```python
from build123d import *

# Parameters (mm, degrees)
F0_W     = 31.8
F0_H     = 15.8
F1_DEPTH = 9.6
F2_R     = 2.4
F3_DEPTH = 1.8
F4_W     = 29.4
F4_H     = 13.4
F5_DEPTH = 8.4
F5_TAPER = 1.5
F6_R     = 1.3
F7_DEPTH = 1.7
F8_R     = 3.25
F8_R_2   = 2.4
F9_DEPTH = 8.4


with BuildPart() as f1:
    # F0 (on Top) → F1 (new body)
    with BuildSketch(Plane.XY):
        Rectangle(F0_W, F0_H)
    extrude(amount=F1_DEPTH)

    # F2 (on face) → F3 (join)
    with BuildSketch(Plane.XY.offset(9.6)):
        with Locations((-12, 4)):
            Circle(F2_R)
        with Locations((-12, -4)):
            Circle(F2_R)
        with Locations((-4, 4)):
            Circle(F2_R)
        with Locations((-4, -4)):
            Circle(F2_R)
        with Locations((4, 4)):
            Circle(F2_R)
        with Locations((4, -4)):
            Circle(F2_R)
        with Locations((12, 4)):
            Circle(F2_R)
        with Locations((12, -4)):
            Circle(F2_R)
    extrude(amount=F3_DEPTH)

    # F4 (on face) → F5 (cut)
    with BuildSketch(Plane(origin=(0, 0, 0), x_dir=(1, 0, 0), z_dir=(0, 0, -1))):
        Rectangle(F4_W, F4_H)
    extrude(amount=-F5_DEPTH, taper=F5_TAPER, mode=Mode.SUBTRACT)

    # F6 (on face) → F7 (cut)
    with BuildSketch(Plane(origin=(0, 0, 8.4), x_dir=(1, 0, 0), z_dir=(0, 0, -1))):
        with Locations((-12, 4)):
            Circle(F6_R)
        with Locations((-4, 4)):
            Circle(F6_R)
        with Locations((4, 4)):
            Circle(F6_R)
        with Locations((12, 4)):
            Circle(F6_R)
        with Locations((12, -4)):
            Circle(F6_R)
        with Locations((4, -4)):
            Circle(F6_R)
        with Locations((-4, -4)):
            Circle(F6_R)
        with Locations((-12, -4)):
            Circle(F6_R)
    extrude(amount=-F7_DEPTH, mode=Mode.SUBTRACT)

    # F8 (on face) → F9 (join, through all)
    with BuildSketch(Plane(origin=(0, 0, 8.4), x_dir=(1, 0, 0), z_dir=(0, 0, -1))):
        Circle(F8_R)
        Circle(F8_R_2, mode=Mode.SUBTRACT)
        with Locations((8, 0)):
            Circle(F8_R)
        with Locations((8, 0)):
            Circle(F8_R_2, mode=Mode.SUBTRACT)
        with Locations((-8, 0)):
            Circle(F8_R)
        with Locations((-8, 0)):
            Circle(F8_R_2, mode=Mode.SUBTRACT)
    extrude(amount=F9_DEPTH)


solid = f1.part
```
Verification items for the finished model (mm, model axes). A direction names the side the tool comes from. Coordinates: 2 decimals unless noted, no trailing zeros. Loops run counter-clockwise (first coordinate to the right, second up) from the corner with the lowest first, then second, coordinate; pieces in that order, holes last. Notation, with made-up numbers: (59, 55) -> (82, 55) arc R23 ccw to (82, 70) -> close; hole circle Ø9 at (52.25, 1). An arc over 180 degrees is marked (long way). Answer in a Markdown table with one row per item.
1) Depth check by flat-ended pin: P1, Ø2.5, axis at x = 12, y = -4, coming from the -Z side; P2, Ø2, axis at x = 12, y = -4.5, coming from the -Z side; P3, Ø6, axis at x = -9, y = 2, coming from the +Z side. Enter the tip coordinate at first touch or a pass-through.
The answers:
| item | result |
|---|---|
| P1 | stops at z = 10.1 |
| P2 | stops at z = 8.4 |
| P3 | stops at z = 11.4 |
2) Draft check along Y on faces 4 (the face through (12, -4, 10.1)), 5 (the face through (15.9, 0, 5)). Enter one of: released by +Y, released by -Y, zero draft, split by the parting line, or undercut.
The answers:
| item | result |
|---|---|
| face 4 | undercut |
| face 5 | zero draft |
3) Section check B-B (z = 5.5). Give the number of separate pieces and of enclosed holes in the cut face, and give its area (3 significant figures).
The answers:
| item | result |
|---|---|
| separate pieces | 4 |
| enclosed holes | 4 |
| area | 166 mm2 |
4) Access from +Z, -Z, +X, -X, +Y, -Y to the whole of each face (thin tool, end or side, straight path). Record for faces 1 (the face through (8, 0, 8.4)), 2 (the face through (-12, -4, 11.4)), 3 (the face through (13.29, 6.024, 10.487)).
The answers:
| item | result |
|---|---|
| face 1 | -Z |
| face 2 | +Z, +X, -X, +Y, -Y |
| face 3 | +Z |
5) Section check A-A (z = 10.5). Record the cut outline in (x, y).
The answers:
| item | result |
|---|---|
| outline | circle Ø4.8 at (-12, -4); circle Ø4.8 at (-12, 4); circle Ø4.8 at (-4, -4); circle Ø4.8 at (-4, 4); circle Ø4.8 at (4, -4); circle Ø4.8 at (4, 4); circle Ø4.8 at (12, -4); circle Ø4.8 at (12, 4) |
6) Scan lines: line 1 along X through (y, z) = (4, 9); line 2 along Y through (x, z) = (-12, 8.85); line 3 along X through (y, z) = (-2.5, 4.75). Record each from-to range of solid material in increasing order. Write a range as from..to.
The answers:
| item | result |
|---|---|
| line 1 | x = -15.9..-13.3, -10.7..-5.3, -2.7..2.7, 5.3..10.7, 13.3..15.9 |
| line 2 | y = -7.9..-5.3, -2.7..2.7, 5.3..7.9 |
| line 3 | x = -15.9..-14.58, -10.08..-5.92, -2.08..2.08, 5.92..10.08, 14.58..15.9 |
